Build history of the part. All positions in model axes, mm. Face numbers are marked on the shaded views. A direction names the side the tool comes from. Give positions to 0.01 mm unless a question says otherwise; leave off trailing zeros. Write each loop counter-clockwise with the first axis right and the second up, starting at its lowest first coordinate (ties: lowest second). Pieces come first, ordered by that corner, then holes. Notation, with made-up numbers: (29.5, 78.25) -> (78.5, 78.25) arc R18 ccw to (78.5, 113.25) -> close; hole circle Ø10 at (85.5, 38). An arc over 180 degrees is marked (long way). Write item = value, one per line. Start each with the question number.
Q1. Saw through at C-C, the plane y = -6.5. List the corners of the cut face in (x, z).
Q2. Saw through at D-D, the plane x = 3.5. List the corners of the cut face in (y, z), then the cut area to 3 significant figures.
Q3. Tool access for the marked faces 1, 2 and 3: list every direction of +Z, -Z, +X, -X, +Y, -Y with a clear straight run to the whole face (end or side of a thin tool).
Q4. Wall check: line 1 (Y direction, x = 7.5, z = 8); line 2 (Z direction, x = 3.5, y = 1); line 3 (X direction, y = -9.75, z = 1). Give the ranges that are in metal, low to high.
Q5. Saw through at A-A, the plane x = 7. List the corners of the cut face in (y, z).
Q6. Mould opens along Z. For the marked faces 4, 5 and 6 say: pulls with the +Z half, pulls with the -Z half, needs draft (parallel to the pull), parting line crosses it, or undercut.
Q7. Drop flat-ended pins along their axis: P1, Ø3, axis at y = -3.5, z = -6.5, coming from the +X side; P2, Ø0.9, axis at y = -1, z = -14.5, coming from the +X side; P3, Ø2.5, axis at x = 6, z = -4.5, coming from the -Y side. Give the stop position or say it passes through.
Q8. Saw through at B-B, the plane z = 6.5. List the corners of the cut face in (x, y), then the cut area to 3 significant figures.
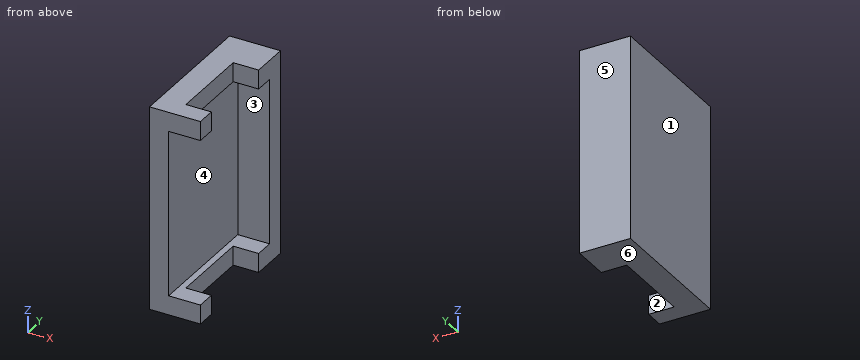
from build123d import *

# Parameters (mm, degrees)
SKETCH1_W           = 32
SKETCH1_H           = 22
BOSS_EXTRUDE1_DEPTH = 3
BOSS_EXTRUDE6_DEPTH = 5
SKETCH8_W           = 4
SKETCH8_H           = 13
CUT_EXTRUDE3_DEPTH  = 32


with BuildPart() as part:
    # Sketch1 → Boss-Extrude1 (new body)
    with BuildSketch(Plane(origin=(0, 0, 0), x_dir=(0, 0, -1), z_dir=(1, 0, 0))):
        Rectangle(SKETCH1_W, SKETCH1_H)
    extrude(amount=BOSS_EXTRUDE1_DEPTH)

    # Sketch7 → Boss-Extrude6 (add)
    with BuildSketch(Plane(origin=(3, 0, 0), x_dir=(0, 0, -1), z_dir=(1, 0, 0))):
        Polygon((16, -11), (16, 11), (-16, 11), (-16, -11), (-13, -11), (-13, 8), (13, 8), (13, -11), align=None)
    extrude(amount=BOSS_EXTRUDE6_DEPTH)

    # Sketch8 → Cut-Extrude3 (cut)
    with BuildSketch(Plane.XY.offset(16)):
        with Locations((6, -1.5)):
            Rectangle(SKETCH8_W, SKETCH8_H)
    extrude(amount=-CUT_EXTRUDE3_DEPTH, mode=Mode.SUBTRACT)


solid = part.part
Report:
q1.outline = (0, -16) -> (4, -16) -> (4, -13) -> (3, -13) -> (3, 13) -> (4, 13) -> (4, 16) -> (0, 16) -> close
q2.outline = (-11, -16) -> (11, -16) -> (11, 16) -> (-11, 16) -> (-11, 13) -> (8, 13) -> (8, -13) -> (-11, -13) -> close
q2.area = 210 mm2
q3.face_1 = +Z, -Z, -X, +Y, -Y
q3.face_2 = +Z, -Z, +X
q3.face_3 = +X, -Y
q4.line_1 = 8 to 11
q4.line_2 = -16 to -13, 13 to 16
q4.line_3 = 0 to 3
q5.outline = (-11, -16) -> (-8, -16) -> (-8, -13) -> (-11, -13) -> close; (-11, 13) -> (-8, 13) -> (-8, 16) -> (-11, 16) -> close; (5, -16) -> (11, -16) -> (11, 16) -> (5, 16) -> (5, 13) -> (8, 13) -> (8, -13) -> (5, -13) -> close
q6.face_4 = undercut
q6.face_5 = needs draft
q6.face_6 = pulls with the -Z half
q7.P1 = 3
q7.P2 = 4
q7.P3 = 8
q8.outline = (0, -11) -> (3, -11) -> (3, 8) -> (8, 8) -> (8, 11) -> (0, 11) -> close
q8.area = 81.0 mm2
